```python
from build123d import *

# Parameters (mm, degrees)
BOSS_EXTRUDE1_DEPTH      = 1.56
CUT_EXTRUDE1_DEPTH       = 1.56
M2_CLEARANCE_HOLE1_D     = 2.4
M2_CLEARANCE_HOLE1_DEPTH = 38.1
M2_CLEARANCE_HOLE1_TIP   = 0.721032743


with BuildPart() as part:
    # Sketch1 → Boss-Extrude1 (new body)
    with BuildSketch(Plane(origin=(0, 0, 0), x_dir=(1, 0, 0), z_dir=(0, 1, 0))):
        with BuildLine():
            Line((-49.356685196, 41.604788024), (-43.256685196, 47.704788024))
            Line((-43.256685196, 47.704788024), (43.143314804, 47.704788024))
            Line((43.143314804, 47.704788024), (49.243314804, 41.604788024))
            Line((49.243314804, 41.604788024), (49.243314804, -37.995211976))
            Line((49.243314804, -37.995211976), (47.743314804, -37.995211976))
            ThreePointArc((47.743314804, -37.995211976), (47.036208023, -38.288105194), (46.743314804, -38.995211976))
            Line((46.743314804, -38.995211976), (46.743314804, -44.095211976))
            ThreePointArc((46.743314804, -44.095211976), (46.450421585, -44.802318757), (45.743314804, -45.095211976))
            Line((45.743314804, -45.095211976), (34.943314804, -45.095211976))
            ThreePointArc((34.943314804, -45.095211976), (34.236208023, -45.388105194), (33.943314804, -46.095211976))
            Line((33.943314804, -46.095211976), (33.943314804, -47.595211976))
            Line((33.943314804, -47.595211976), (-34.056685196, -47.595211976))
            Line((-34.056685196, -47.595211976), (-34.056685196, -46.095211976))
            ThreePointArc((-34.056685196, -46.095211976), (-34.349578415, -45.388105194), (-35.056685196, -45.095211976))
            Line((-35.056685196, -45.095211976), (-45.856685196, -45.095211976))
            ThreePointArc((-45.856685196, -45.095211976), (-46.563791977, -44.802318757), (-46.856685196, -44.095211976))
            Line((-46.856685196, -44.095211976), (-46.856685196, -38.995211976))
            ThreePointArc((-46.856685196, -38.995211976), (-47.149578415, -38.288105194), (-47.856685196, -37.995211976))
            Line((-47.856685196, -37.995211976), (-49.356685196, -37.995211976))
            Line((-49.356685196, -37.995211976), (-49.356685196, 41.604788024))
        make_face()
    extrude(amount=BOSS_EXTRUDE1_DEPTH)

    # Sketch2 → Cut-Extrude1 (cut)
    with BuildSketch(Plane(origin=(0, 1.56, 0), x_dir=(1, 0, 0), z_dir=(0, 1, 0))):
        Polygon((-40.243314804, 31.704788024), (-33.243314804, 38.704788024), (33.243314804, 38.704788024), (40.243314804, 31.704788024), (40.243314804, -31.704788024), (33.243314804, -38.704788024), (-33.243314804, -38.704788024), (-40.243314804, -31.704788024), align=None)
    extrude(amount=-CUT_EXTRUDE1_DEPTH, mode=Mode.SUBTRACT)

    # M2 Clearance Hole1
    with Locations(Plane(origin=(0, 1.56, 0), x_dir=(1, 0, 0), z_dir=(0, 1, 0))):
        with Locations((40.929491149, 39.39737116), (40.929491149, -39.39737116), (-40.929491149, -39.39737116), (-40.929491149, 39.39737116), (0, 0)):
            Hole(M2_CLEARANCE_HOLE1_D / 2, depth=M2_CLEARANCE_HOLE1_DEPTH)
            with Locations((0, 0, -(M2_CLEARANCE_HOLE1_DEPTH + M2_CLEARANCE_HOLE1_TIP / 2))):  # 118° drill point
                Cone(0, M2_CLEARANCE_HOLE1_D / 2, M2_CLEARANCE_HOLE1_TIP, mode=Mode.SUBTRACT)


solid = part.part
```
The model under review builds one solid part; all positions refer to its coordinate system, in mm. A direction names the side the tool comes from. Coordinates: 2 decimals unless noted, no trailing zeros. Loops run counter-clockwise (first coordinate to the right, second up) from the corner with the lowest first, then second, coordinate; pieces in that order, holes last. Notation, with made-up numbers: (71, 64.25) -> (116, 64.25) arc R30 ccw to (116, 103.25) -> close; hole circle Ø7 at (82.5, -5). An arc over 180 degrees is marked (long way). Answer as CSV lines item,"result".
Item 1: Machinability: for faces 1 (the flat face through (-36.694, 0.791, 35.254)), 2 (the flat face through (46.15, 0.77, -44.7)), which of the approach directions +Z, -Z, +X, -X, +Y, -Y give a long, thin tool a straight path to every point of the face, cutting with its end or side? Answer none if there is none.
Results below:
face 1,"+Y, -Y"
face 2,"-Z, +X, +Y, -Y"
Item 2: Take a section at C-C, the plane y = 1.1. Count the separate pieces of the cut face and the enclosed holes in it, and give its area (3 significant figures).
Results below:
separate pieces,"1"
enclosed holes,"5"
area,"3,100 mm2"
Item 3: Draft analysis for pull direction X (two halves, no side actions). For faces 3 (the cylindrical face through (40.38, 0.77, -38.33)), 4 (the flat face through (-36.79, 0.79, -35.16)), 5 (the flat face through (-46.35, 0.77, -44.61)), 6 (the flat face through (1, 0, 42)), state which applies: +X half, -X half, draft (parallel to the pull), parting line (faces both ways), or undercut.
Results below:
face 3,"undercut"
face 4,"undercut"
face 5,"-X half"
face 6,"draft"
Item 4: Insertion check: pin 1 (0.8 mm diameter, centred on y = 1, z = 46.5, fed in from +X); pin 2 (0.8 mm diameter, centred on x = 42.5, y = 0.5, fed in from +Z); pin 3 (0.8 mm diameter, centred on y = 1, z = 43, fed in from +X); pin 4 (3 mm diameter, centred on x = 40.93, z = -39.4, fed in from -Y). Each pin has a flat end and moves straight along its axis. Give the tip position at first contact, or say it passes through.
Results below:
pin 1,"stops at x = 33.94"
pin 2,"stops at z = 45.1"
pin 3,"stops at x = 46.74"
pin 4,"stops at y = 0"
Item 5: Take a section at B-B, the plane x = -10.5. State the section outline as (y, z) points, and give its area (3 significant figures).
Results below:
outline,"(0, -47.7) -> (1.56, -47.7) -> (1.56, -38.7) -> (0, -38.7) -> close; (0, 38.7) -> (1.56, 38.7) -> (1.56, 47.6) -> (0, 47.6) -> close"
area,"27.9 mm2"
Item 6: For L1, parallel to X at y = 0.4, z = -28.5; L2, parallel to Z at x = -29.5, y = 0.7; L3, parallel to Z at x = 44, y = 0.55, list the stretches that pass through material, from the lowest coordinate up.
Results below:
L1,"x = -49.36 to -40.24, 40.24 to 49.24"
L2,"z = -47.7 to -38.7, 38.7 to 47.6"
L3,"z = -46.85 to 45.1"
Item 7: Take a section at A-A, the plane z = 8. State the section outline as (x, y) points.
Results below:
outline,"(-49.36, 0) -> (-40.24, 0) -> (-40.24, 1.56) -> (-49.36, 1.56) -> close; (40.24, 0) -> (49.24, 0) -> (49.24, 1.56) -> (40.24, 1.56) -> close"
Item 8: Take a section at D-D, the plane z = 42.5. State the section outline as (x, y) points, and give its area (3 significant figures).
Results below:
outline,"(-46.86, 0) -> (46.74, 0) -> (46.74, 1.56) -> (-46.86, 1.56) -> close"
area,"146 mm2"
